from build123d import *

# Parameters (mm, degrees)
SKETCH1_R           = 3
SKETCH1_R_2         = 1
BOSS_EXTRUDE1_DEPTH = 1.5
CUT_EXTRUDE1_DEPTH  = 2


with BuildPart() as part:
    # Sketch1 → Boss-Extrude1 (new body, symmetric)
    with BuildSketch(Plane(origin=(0, 0, 0), x_dir=(0, 0, -1), z_dir=(1, 0, 0))):
        Circle(SKETCH1_R)
        Circle(SKETCH1_R_2, mode=Mode.SUBTRACT)
    extrude(amount=BOSS_EXTRUDE1_DEPTH, both=True)

    # Sketch2 → Cut-Extrude1 (cut)
    with BuildSketch(Plane.ZY.offset(1.5)):
        with BuildLine():
            Line((2, -2.236067977), (2, 2.236067977))
            ThreePointArc((2, 2.236067977), (-1.224744871, 2.738612788), (-3, 0))
            Line((-3, 0), (-1, 0))
            ThreePointArc((-1, 0), (0, 1), (1, 0))
            ThreePointArc((1, 0), (0.707106781, -0.707106781), (0, -1))
            Line((0, -1), (0, -3))
            ThreePointArc((0, -3), (1.070466269, -2.802517077), (2, -2.236067977))
        make_face()
    extrude(amount=-CUT_EXTRUDE1_DEPTH, mode=Mode.SUBTRACT)


solid = part.part
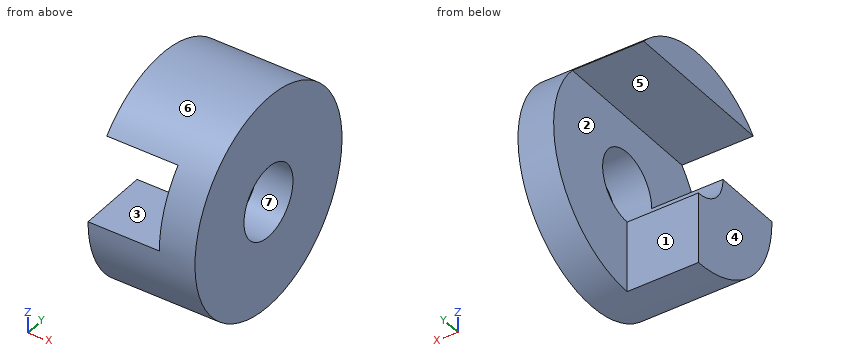
Geometry: final body of the model. Coordinates: model frame, mm. Face numbers are marked on the shaded views. A direction names the side the tool comes from. Round coordinates to 2 decimals unless told otherwise and drop trailing zeros. Loops run counter-clockwise (first coordinate to the right, second up) from the corner with the lowest first, then second, coordinate; pieces in that order, holes last. Notation, with made-up numbers: (-5, 58) - (42, 58) arc R19 ccw to (42, 78) - close; hole circle Ø7 at (39, -12.75). An arc over 180 degrees is marked (long way). Write each question's results on one line, items separated by ' | '. Start each with the question number.
1) Line query: probe 1 along X at (y, z) = (2, -0.75); probe 2 along Y at (x, z) = (-0.45, -2); probe 3 along Z at (x, y) = (-0.65, -0.5). Output: solid intervals per line, ascending. Write a range as [from, to].
2) Cut plane A-A on x = -0.55. Return loops of the section in (y, z).
3) Cut plane C-C on z = -0.5. Return loops of the section in (x, y).
4) Mould query, pull axis Y, two halves, no side actions, for the marked faces 5, 6 and 7. Classes: released by +Y, released by -Y, zero draft, split by the parting line, or undercut.
5) Cut plane B-B on y = -0.75. Return loops of the section in (x, z), then the cut area to 3 significant figures.
6) Cut plane D-D on y = -2. Return loops of the section in (x, z), then the cut area to 3 significant figures.
7) Access query for the marked faces 1, 2, 3 and 4. Directions: +Z, -Z, +X, -X, +Y, -Y. A direction counts if a zero-diameter tool reaches every point of the face in a straight line with its end or side. Return the directions, or none.
Verdict:
1) probe 1: x = [0.5, 1.5] | probe 2: y = [-2.24, 0] | probe 3: z = [-2.96, -0.87], [2, 2.96]
2) outline: (-3, 0) arc R3 ccw to (0, -3) - (0, -1) arc R1 cw to (-1, 0) - close; (-2.24, 2) - (2.24, 2) arc R3 ccw to start
3) outline: (-1.5, -2.96) - (1.5, -2.96) - (1.5, -0.87) - (-1.5, -0.87) - close; (0.5, 0.87) - (1.5, 0.87) - (1.5, 2.96) - (0.5, 2.96) - close
4) face 5: zero draft | face 6: split by the parting line | face 7: undercut
5) outline: (-1.5, -2.9) - (1.5, -2.9) - (1.5, -0.66) - (-1.5, -0.66) - close; (-1.5, 2) - (0.5, 2) - (0.5, 0.66) - (1.5, 0.66) - (1.5, 2.9) - (-1.5, 2.9) - close | area: 10.8 mm2
6) outline: (-1.5, -2.24) - (1.5, -2.24) - (1.5, 2.24) - (-1.5, 2.24) - (-1.5, 2) - (0.5, 2) - (0.5, 0) - (-1.5, 0) - close | area: 9.42 mm2
7) face 1: -Z, -X, +Y | face 2: -X, +Y | face 3: -X, +Y, -Y | face 4: +Z, -Z, -X, +Y, -Y
